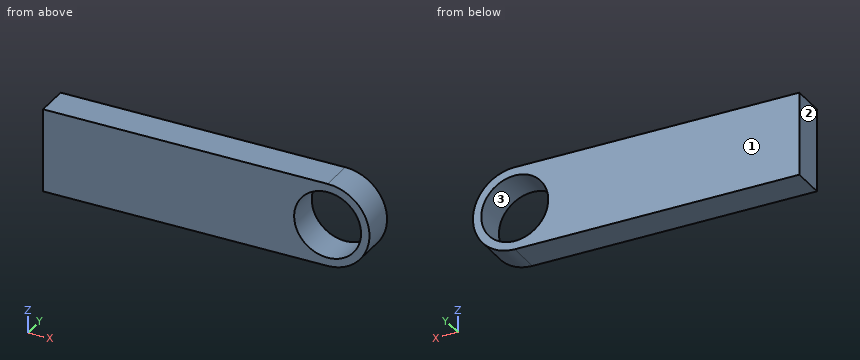
from build123d import *

# Parameters (mm, degrees)
EXTRUDE_1_DEPTH     = 2
SKETCH_2_R          = 2
CUT_EXTRUDE_1_DEPTH = 3


with BuildPart() as part:
    # Эскиз1 → Бобышка-Вытянуть1 (new body)
    with BuildSketch(Plane(origin=(0, 0, 0), x_dir=(1, 0, 0), z_dir=(0, 1, 0))):
        with BuildLine():
            Line((0, 2.5), (-17, 2.5))
            Line((-17, 2.5), (-17, -2.5))
            Line((-17, -2.5), (0, -2.5))
            ThreePointArc((0, -2.5), (2.5, 0), (0, 2.5))
        make_face()
    extrude(amount=EXTRUDE_1_DEPTH)

    # Эскиз2 → Вырез-Вытянуть1 (cut)
    with BuildSketch(Plane(origin=(0, 2, 0), x_dir=(1, 0, 0), z_dir=(0, 1, 0))):
        with Locations(Location((0, 0, 0), (0, 0, 270))):
            Circle(SKETCH_2_R)
    extrude(amount=-CUT_EXTRUDE_1_DEPTH, mode=Mode.SUBTRACT)


solid = part.part
Source: CAD feature listing. Evaluate the final solid. Frame: model axes, mm. Face numbers are marked on the shaded views. Give positions to 0.01 mm unless a question says otherwise; leave off trailing zeros. Write each loop counter-clockwise with the first axis right and the second up, starting at its lowest first coordinate (ties: lowest second). Pieces come first, ordered by that corner, then holes. Notation, with made-up numbers: M 51,-37 L 103,-37 A31 cw 103,-7 Z; hole C -30,50.5 d10. An arc over 180 degrees is marked long. Return JSON: item names as keys, results as strings. Group by question number.
1) Ray query, L1, parallel to X at y = 1.5, z = 0; L2, parallel to X at y = 0.7, z = 1.6; L3, parallel to X at y = 1, z = 2.15. Return the intervals inside material, ascending.
2) Draft query along X for the marked faces 1, 2 and 3. Return one class per face: released by +X, released by -X, zero draft, split by the parting line, or undercut.
3) Cut plane C-C, the plane y = 1.05. Output: boundary loops of the cut face in (x, z), then the cut area to 3 significant figures.
4) Cut plane A-A, the plane z = 0. Output: boundary loops of the cut face in (x, y), then the cut area to 3 significant figures.
5) Cut plane B-B, the plane x = -0.5. Output: boundary loops of the cut face in (y, z), then the cut area to 3 significant figures.
Data:
{
 "1": {"L1": "x = -17 to -2, 2 to 2.5", "L2": "x = -17 to -1.2, 1.2 to 1.92", "L3": "x = -17 to 1.28"},
 "2": {"face 1": "zero draft", "face 2": "released by -X", "face 3": "undercut"},
 "3": {"outline": "M -17,-2.5 L 0,-2.5 A2.5 ccw 0,2.5 L -17,2.5 Z; hole C 0,0 d4", "area": "82.3 mm²"},
 "4": {"outline": "M -17,0 L -2,0 L -2,2 L -17,2 Z; M 2,0 L 2.5,0 L 2.5,2 L 2,2 Z", "area": "31.0 mm²"},
 "5": {"outline": "M 0,-2.5 L 2,-2.5 L 2,-1.94 L 0,-1.94 Z; M 0,1.94 L 2,1.94 L 2,2.5 L 0,2.5 Z", "area": "2.25 mm²"}
}
